The listing builds one solid part. Answer for the finished solid, in the listing's coordinates (mm). Face numbers are marked on the shaded views. A direction names the side the tool comes from. Coordinates: 2 decimals unless noted, no trailing zeros. Loops run counter-clockwise (first coordinate to the right, second up) from the corner with the lowest first, then second, coordinate; pieces in that order, holes last. Notation, with made-up numbers: (52, 53) - (61, 53) arc R16 cw to (61, 57) - close; hole circle Ø8 at (75.25, 89). An arc over 180 degrees is marked (long way). Put each result on its own line as item: value.
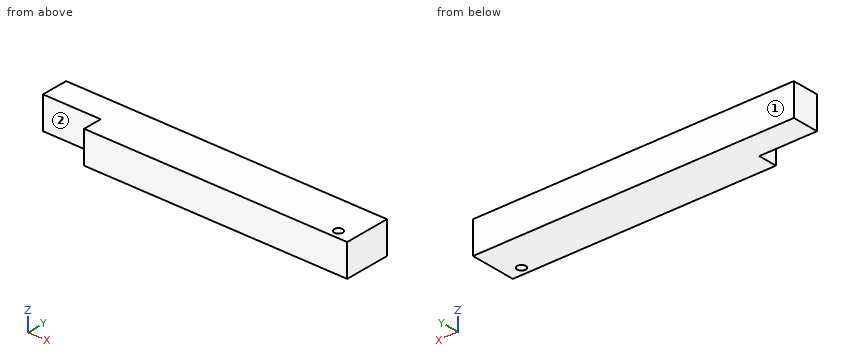
```python
from build123d import *

# Parameters (mm, degrees)
ESQUISSE1_W                  = 300
ESQUISSE1_H                  = 25
BOSS_EXTRU_1_DEPTH           = 30
ESQUISSE3_W                  = 246
ESQUISSE3_H                  = 18
BOSS_EXTRU_2_DEPTH           = 30
ENL_V_MAT_EXTRU_1_DEPTH      = 303.530990148
ENL_V_MAT_EXTRU_1_DEPTH_BACK = 303.530990148
ESQUISSE2_R                  = 4


with BuildPart() as part:
    # Esquisse1 → Boss.-Extru.1 (new body)
    with BuildSketch(Plane.XY):
        with Locations((150, 12.5)):
            Rectangle(ESQUISSE1_W, ESQUISSE1_H)
    extrude(amount=BOSS_EXTRU_1_DEPTH)

    # Esquisse3 → Boss.-Extru.2 (add)
    with BuildSketch(Plane.XY.offset(30)):
        with Locations((177, -9)):
            Rectangle(ESQUISSE3_W, ESQUISSE3_H)
    extrude(amount=-BOSS_EXTRU_2_DEPTH)

    # Esquisse2 → Enlèv. mat.-Extru.1 (cut, two sides: drawn at the far end of the back side and taken through both)
    with BuildSketch(Plane.XY.offset(30).offset(-ENL_V_MAT_EXTRU_1_DEPTH_BACK)):
        with Locations((285, -10)):
            Circle(ESQUISSE2_R)
    extrude(amount=ENL_V_MAT_EXTRU_1_DEPTH + ENL_V_MAT_EXTRU_1_DEPTH_BACK, mode=Mode.SUBTRACT)


solid = part.part
```
1) The part is cut by section D-D (x = 41). Give the vertices of the cut face in (y, z), and give its area (3 significant figures).
Found:
outline: (0, 0) - (25, 0) - (25, 30) - (0, 30) - close
area: 750 mm^2
2) Straight lines are drawn through the part: L1, parallel to X at y = -10, z = 16.75; L2, parallel to Y at x = 285, z = 9; L3, parallel to X at y = -14.5, z = 18. For each, find the intervals that lie inside material, in ascending order. Write a range as [from, to].
Found:
L1: x = [54, 281], [289, 300]
L2: y = [-18, -14], [-6, 25]
L3: x = [54, 300]
3) The part is cut by section B-B (z = 13.5). Give the vertices of the cut face in (x, y).
Found:
outline: (0, 0) - (54, 0) - (54, -18) - (300, -18) - (300, 25) - (0, 25) - close; hole circle Ø8 at (285, -10)
4) The part is cut by section C-C (y = -10). Give the vertices of the cut face in (x, z), and give its area (3 significant figures).
Found:
outline: (54, 0) - (281, 0) - (281, 30) - (54, 30) - close; (289, 0) - (300, 0) - (300, 30) - (289, 30) - close
area: 7,140 mm^2
5) For the marked faces 1 and 2, determine the directions among +Z, -Z, +X, -X, +Y, -Y from which every point of the face is accessible in a straight line to the end or side of a thin tool.
Found:
face 1: +Z, -Z, +X, -X, +Y
face 2: +Z, -Z, -X, -Y
6) The part is cut by section A-A (x = 285). Give the vertices of the cut face in (y, z), and give its area (3 significant figures).
Found:
outline: (-18, 0) - (-14, 0) - (-14, 30) - (-18, 30) - close; (-6, 0) - (25, 0) - (25, 30) - (-6, 30) - close
area: 1,050 mm^2
7) This flat-tipped pin is pushed along its axis until it touches: pin 1 (5.5 mm diameter, centred on y = -9.5, z = 12, fed in from -X). Where does it stop, or does it pass through?
Found:
pin 1: stops at x = 54
